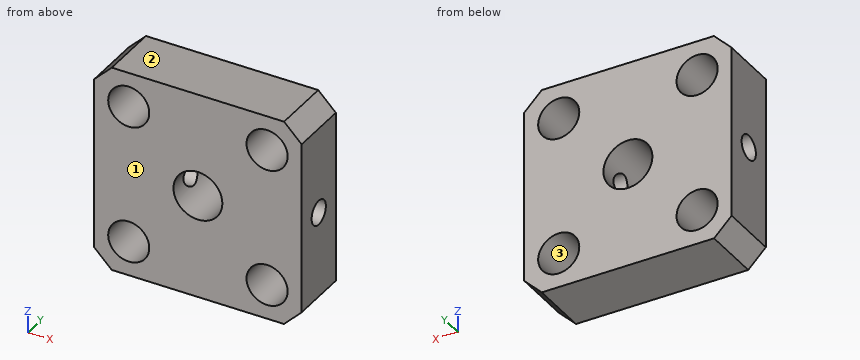
from build123d import *

# Parameters (mm, degrees)
SKETCH1_W             = 21.21
SKETCH1_H             = 21.21
SKETCH1_R             = 2.5
BOSS_EXTRUDE1_DEPTH   = 6
M5X0_8_TAPPED_HOLE1_D = 4.2
M3X0_5_TAPPED_HOLE1_D = 2.5
CHAMFER1_SIZE         = 1.8


with BuildPart() as part:
    # Sketch1 → Boss-Extrude1 (new body)
    with BuildSketch(Plane(origin=(0, 0, 0), x_dir=(1, 0, 0), z_dir=(0, 1, 0))):
        Rectangle(SKETCH1_W, SKETCH1_H)
        Circle(SKETCH1_R, mode=Mode.SUBTRACT)
    extrude(amount=BOSS_EXTRUDE1_DEPTH)

    # M5x0.8 Tapped Hole1 (through all)
    with Locations(Plane(origin=(0, 6, 0), x_dir=(1, 0, 0), z_dir=(0, 1, 0))):
        with Locations((-7.071067812, 7.071067812), (-7.071067812, -7.071067812), (7.071067812, -7.071067812), (7.071067812, 7.071067812)):
            Hole(M5X0_8_TAPPED_HOLE1_D / 2)

    # M3x0.5 Tapped Hole1 (through all)
    with Locations(Plane(origin=(10.605, 0, 0), x_dir=(0, 0, -1), z_dir=(1, 0, 0))):
        with Locations((0, 3)):
            Hole(M3X0_5_TAPPED_HOLE1_D / 2)

    # Chamfer1
    chamfer1_edges = [part.edges().sort_by_distance(p)[0] for p in [
        (-10.605, 3, -10.605),
        (10.605, 3, -10.605),
        (10.605, 3, 10.605),
        (-10.605, 3, 10.605),
    ]]
    chamfer(chamfer1_edges, length=CHAMFER1_SIZE)


solid = part.part
Here's how the part is built. I have some questions about the finished solid (model axes, mm). Face numbers are marked on the shaded views. Round coordinates to 2 decimals unless told otherwise and drop trailing zeros. Write each loop counter-clockwise with the first axis right and the second up, starting at its lowest first coordinate (ties: lowest second). Pieces come first, ordered by that corner, then holes.
1. I need wall thicknesses on L1, parallel to X at y = 2, z = -9; L2, parallel to Z at x = 0, y = 3.75 (3 decimals); L3, parallel to X at y = 1.5, z = -1.25 (3 decimals). Which ranges of each line are inside material? Lowest first, please.
2. If we mould it in two halves opening along Z, with no side actions, what happens to the marked faces 1, 2 and 3? For each: released by +Z, released by -Z, zero draft, split by the parting line, or undercut.
3. Suppose I cut it at D-D (x = 3.75). List the corners of the cut face in (y, z) for me (3 decimals).
4. Suppose I cut it at C-C (y = 2.5). List the corners of the cut face in (x, z) for me (3 decimals), and give its area (3 significant figures).
5. Suppose I cut it at B-B (x = -6). List the corners of the cut face in (y, z) for me (3 decimals).
6. Suppose I cut it at A-A (z = 0). List the corners of the cut face in (x, y) for me (3 decimals), and give its area (3 significant figures).
Answer sheet:
1. L1: x = -10.41 to -7.9, -6.24 to 6.24, 7.9 to 10.41
1. L2: z = -10.605 to -2.5, 2.5 to 10.605
1. L3: x = -10.605 to -2.165, 2.165 to 10.605
2. face 1: zero draft
2. face 2: released by +Z
2. face 3: undercut
3. outline: (0, -10.605) - (6, -10.605) - (6, 10.605) - (0, 10.605) - close; hole circle Ø2.5 at (3, 0)
4. outline: (-10.605, -8.805) - (-8.805, -10.605) - (8.805, -10.605) - (10.605, -8.805) - (10.605, -1.146) - (2.222, -1.146) arc R2.5 cw to (-2.222, -1.146) - (-10.605, -1.146) - close; (-10.605, 1.146) - (-2.222, 1.146) arc R2.5 cw to (2.222, 1.146) - (10.605, 1.146) - (10.605, 8.805) - (8.805, 10.605) - (-8.805, 10.605) - (-10.605, 8.805) - close; hole circle Ø4.2 at (-7.071, -7.071); hole circle Ø4.2 at (-7.071, 7.071); hole circle Ø4.2 at (7.071, -7.071); hole circle Ø4.2 at (7.071, 7.071)
4. area: 331 mm2
5. outline: (0, -10.605) - (6, -10.605) - (6, -8.877) - (0, -8.877) - close; (0, -5.265) - (6, -5.265) - (6, 5.265) - (0, 5.265) - close; (0, 8.877) - (6, 8.877) - (6, 10.605) - (0, 10.605) - close; hole circle Ø2.5 at (3, 0)
6. outline: (-10.605, 0) - (-2.5, 0) - (-2.5, 1.75) - (-10.605, 1.75) - close; (-10.605, 4.25) - (-2.5, 4.25) - (-2.5, 6) - (-10.605, 6) - close; (2.5, 0) - (10.605, 0) - (10.605, 1.75) - (2.5, 1.75) - close; (2.5, 4.25) - (10.605, 4.25) - (10.605, 6) - (2.5, 6) - close
6. area: 56.7 mm2
